The listing builds one solid part. Answer for the finished solid, in the listing's coordinates (mm). Face numbers are marked on the shaded views. A direction names the side the tool comes from. Round coordinates to 2 decimals unless told otherwise and drop trailing zeros. Write each loop counter-clockwise with the first axis right and the second up, starting at its lowest first coordinate (ties: lowest second). Pieces come first, ordered by that corner, then holes.
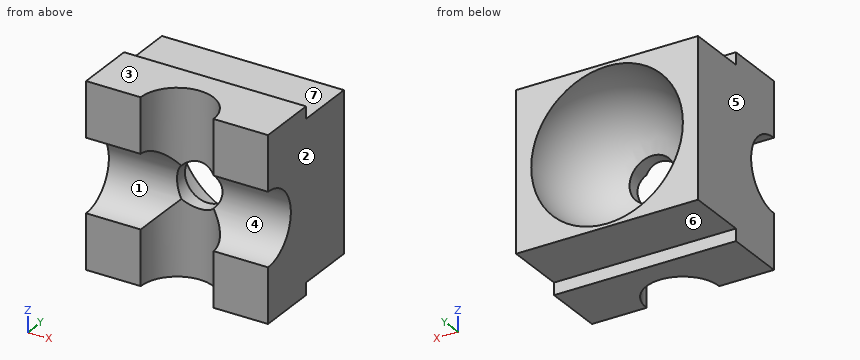
from build123d import *

# Parameters (mm, degrees)
SKETCH2_W               = 30
SKETCH2_H               = 30
BOSS_EXTRUDE1_DEPTH     = 20
SKETCH3_R               = 6
CUT_EXTRUDE2_DEPTH      = 1
CUT_EXTRUDE2_DEPTH_BACK = 31
SKETCH4_R               = 6
CUT_EXTRUDE3_DEPTH      = 1
CUT_EXTRUDE3_DEPTH_BACK = 31
SKETCH7_R               = 3.75
CUT_EXTRUDE4_DEPTH      = 21
SKETCH8_W               = 30
SKETCH8_H               = 10
CUT_EXTRUDE6_DEPTH      = 2
SKETCH9_W               = 30
SKETCH9_H               = 10
CUT_EXTRUDE7_DEPTH      = 2


with BuildPart() as part:
    # Sketch2 → Boss-Extrude1 (new body)
    with BuildSketch(Plane(origin=(0, 0, 0), x_dir=(1, 0, 0), z_dir=(0, 1, 0))):
        Rectangle(SKETCH2_W, SKETCH2_H)
    extrude(amount=BOSS_EXTRUDE1_DEPTH)

    # Sketch3 → Cut-Extrude2 (cut, two sides)
    with BuildSketch(Plane.XY.offset(15)) as cut_extrude2_sk:
        Circle(SKETCH3_R)
    extrude(amount=CUT_EXTRUDE2_DEPTH, mode=Mode.SUBTRACT)
    extrude(cut_extrude2_sk.sketch, amount=-CUT_EXTRUDE2_DEPTH_BACK, mode=Mode.SUBTRACT)

    # Sketch4 → Cut-Extrude3 (cut, two sides)
    with BuildSketch(Plane(origin=(15, 0, 0), x_dir=(0, 0, -1), z_dir=(1, 0, 0))) as cut_extrude3_sk:
        Circle(SKETCH4_R)
    extrude(amount=CUT_EXTRUDE3_DEPTH, mode=Mode.SUBTRACT)
    extrude(cut_extrude3_sk.sketch, amount=-CUT_EXTRUDE3_DEPTH_BACK, mode=Mode.SUBTRACT)

    # Sketch5 → Cut-Revolve1 (revolve, cut)
    with BuildSketch(Plane(origin=(0, 20, 0), x_dir=(1, 0, 0), z_dir=(0, 1, 0))):
        with BuildLine():
            Line((12.5, 0), (-12.5, 0))
            ThreePointArc((-12.5, 0), (0, 12.5), (12.5, 0))
        make_face()
    revolve(axis=Axis((12.5, 20, 0), (-1, 0, 0)), mode=Mode.SUBTRACT)

    # Sketch7 → Cut-Extrude4 (cut, through all)
    with BuildSketch(Plane(origin=(0, 20, 0), x_dir=(1, 0, 0), z_dir=(0, 1, 0))):
        Circle(SKETCH7_R)
    extrude(amount=-CUT_EXTRUDE4_DEPTH, mode=Mode.SUBTRACT)

    # Sketch8 → Cut-Extrude6 (cut)
    with BuildSketch(Plane.XY.offset(15)):
        with Locations((0, 15)):
            Rectangle(SKETCH8_W, SKETCH8_H)
    extrude(amount=-CUT_EXTRUDE6_DEPTH, mode=Mode.SUBTRACT)

    # Sketch9 → Cut-Extrude7 (cut)
    with BuildSketch(Plane(origin=(0, 0, -15), x_dir=(-1, 0, 0), z_dir=(0, 0, -1))):
        with Locations((0, 15)):
            Rectangle(SKETCH9_W, SKETCH9_H)
    extrude(amount=-CUT_EXTRUDE7_DEPTH, mode=Mode.SUBTRACT)


solid = part.part
1. A tool of negligible diameter and unlimited length cuts with its end or side. For the marked faces 5, 6 and 7, from which of +Z, -Z, +X, -X, +Y, -Y can it reach the whole face along a straight path? Write none if from no direction.
Geometry says:
face 5: +Z, -Z, -X, +Y, -Y
face 6: -Z, +X, -X, +Y
face 7: +Z, +X, -X, +Y
2. Straight lines are drawn through the part: line 1 along X through (y, z) = (7.25, 0); line 2 along Z through (x, y) = (3, 10.25); line 3 along Z through (x, y) = (-9.5, 13.5). For each, find the intervals that lie inside material, in ascending order.
Geometry says:
line 1: x = -15 to -3.75, 3.75 to 15
line 2: z = -13 to -7.22, 7.22 to 13
line 3: z = -13 to -4.87, 4.87 to 13
3. Section A-A on z = 0 is taken. Determine the outline of the cut face in (x, y).
Geometry says:
outline: (-15, 6) - (-3.75, 6) - (-3.75, 8.08) arc R12.5 cw to (-12.5, 20) - (-15, 20) - close; (3.75, 6) - (15, 6) - (15, 20) - (12.5, 20) arc R12.5 cw to (3.75, 8.08) - close
4. Section C-C on y = 6.5 is taken. Determine the outline of the cut face in (x, z).
Geometry says:
outline: (-15, -15) - (15, -15) - (15, 15) - (-15, 15) - close; hole circle Ø7.5 at (0, 0)
5. Section B-B on x = 0 is taken. Determine the outline of the cut face in (y, z), plus the area to 3 significant figures.
Geometry says:
outline: (6, -15) - (10, -15) - (10, -13) - (20, -13) - (20, -12.5) arc R12.5 cw to (8.08, -3.75) - (6, -3.75) - close; (6, 3.75) - (8.08, 3.75) arc R12.5 cw to (20, 12.5) - (20, 13) - (10, 13) - (10, 15) - (6, 15) - close
area: 122 mm2
6. Section D-D on x = 13 is taken. Determine the outline of the cut face in (y, z).
Geometry says:
outline: (0, -15) - (10, -15) - (10, -13) - (20, -13) - (20, 13) - (10, 13) - (10, 15) - (0, 15) - (0, 6) arc R6 cw to (0, -6) - close
7. For a pull along Z with two mould halves and no side action, classify the marked faces 1, 2, 3 and 4 as released by +Z, released by -Z, zero draft, split by the parting line, or undercut.
Geometry says:
face 1: undercut
face 2: zero draft
face 3: released by +Z
face 4: undercut
8. Given pin 1 (5 mm diameter, centred on x = 2.5, y = 16, fed in from +Z); pin 2 (1 mm diameter, centred on x = -4.5, z = 14.5, fed in from +Y); pin 3 (3 mm diameter, centred on x = -3.5, y = 13, fed in from -Z), each flat-ended and moving along its own axis, determine where each tip first touches the part or whether it passes through.
Geometry says:
pin 1: stops at z = 13
pin 2: stops at y = 10
pin 3: stops at z = -13
